from build123d import *

# Parameters (mm, degrees)
F0_R     = 8.5
F0_R_2   = 7
F1_DEPTH = 6.6
F0_R_3   = 3.1
F2_DEPTH = 9
F3_R     = 8.5
F3_R_2   = 7
F3_R_3   = 3.1
F4_DEPTH = 5
F0_R_4   = 2.6
F5_DEPTH = 6.2
F6_SIZE  = 1
F7_SIZE2 = 4
F7_SIZE  = 6
F8_SIZE  = 0.74999


# Not quite as in the source:
# - a fillet or chamfer is up to 0.001 mm smaller than in the source, because OpenCascade refuses the exact size


with BuildPart() as f1:
    # F0 (on Top) → F1 (new body)
    with BuildSketch(Plane.XY):
        Circle(F0_R)
        Circle(F0_R_2, mode=Mode.SUBTRACT)
    extrude(amount=F1_DEPTH)

    # F0 (on Top) → F2 (join)
    with BuildSketch(Plane.XY):
        Circle(F0_R_2)
        Circle(F0_R_3, mode=Mode.SUBTRACT)
    extrude(amount=F2_DEPTH)

    # F3 (on face) → F4 (join)
    with BuildSketch(Plane.XY.offset(9)):
        Circle(F3_R)
        Circle(F3_R_2, mode=Mode.SUBTRACT)
        Circle(F3_R_2)
        Circle(F3_R_3, mode=Mode.SUBTRACT)
    extrude(amount=F4_DEPTH)

    # F0 (on Top) → F5 (join)
    with BuildSketch(Plane.XY):
        Circle(F0_R_3)
        Circle(F0_R_4, mode=Mode.SUBTRACT)
    extrude(amount=F5_DEPTH)

    # F6
    f6_edges = [f1.edges().sort_by_distance(p)[0] for p in [
        (-2.6, 0, 0),
        (-8.5, 0, 0),
    ]]
    chamfer(f6_edges, length=F6_SIZE)

    # F7
    f7_edges = [f1.edges().sort_by_distance(p)[0] for p in [
        (-3.1, 0, 14),
    ]]
    f7_side = f1.faces().sort_by_distance((-3.1, 0, 10.1))[0]
    chamfer(f7_edges, length=F7_SIZE, length2=F7_SIZE2, reference=f7_side)

    # F8 (size 0.75 in the source; OpenCascade refuses exactly that, so slightly less here)
    f8_edges = [f1.edges().sort_by_distance(p)[0] for p in [
        (-7, 0, 9),
        (-7, 0, 6.6),
        (-8.5, 0, 6.6),
        (-8.5, 0, 9),
    ]]
    chamfer(f8_edges, length=F8_SIZE)


solid = f1.part
Build history of the part. All positions in model axes, mm. A direction names the side the tool comes from. Give positions to 0.01 mm unless a question says otherwise; leave off trailing zeros. Order: outer loops, then holes, each group sorted by start corner. A loop starts at its lowest first (then second) coordinate and runs counter-clockwise, first axis right, second up. Notation, with made-up numbers: M -30.5,-29.5 L -10.5,-29.5 A12 ccw -10.5,-14.5 Z; hole C -29,30 d7. An arc over 180 degrees is marked long. Put each result on its own line as item: value.
Item 1: Drop flat-ended pins along their axis: pin 1 Ø3 at (x, z) = (-3, 7.5) entering from +Y; pin 2 Ø4.5 at (x, y) = (1.5, -3) entering from -Z; pin 3 Ø5.5 at (x, y) = (0, 0) entering from +Z; pin 4 Ø8 at (y, z) = (-4.5, 5.5) entering from -X. Give the stop position or say it passes through.
Results are:
pin 1: y = 7.88
pin 2: z = 0
pin 3: z = 6.2
pin 4: x = -8.49
Item 2: Wall check: probe 1 along Y at (x, z) = (0, 2.85); probe 2 along Y at (x, z) = (0, 7.6); probe 3 along X at (y, z) = (-2.5, 11.5). Give the ranges that are in metal, low to high.
Results are:
probe 1: -8.5 to -2.6, 2.6 to 8.5
probe 2: -7 to -3.1, 3.1 to 7
probe 3: -8.12 to -4.82, 4.82 to 8.12
Item 3: Pull direction Y, two halves, no side cores. Call faces 3 (the face through (-0.338, 2.578, 3.564)), 4 (the face through (6.466, -2.681, 7.794)), 5 (the face through (-2, -7, 14)), 6 (the face through (-2, -2, 6.2)): +Y half, -Y half, draft (parallel to the pull), parting line (faces both ways), or undercut.
Results are:
face 3: undercut
face 4: parting line
face 5: draft
face 6: undercut
Item 4: Which spindle directions (+Z, -Z, +X, -X, +Y, -Y) get a long thin tool onto all of the face, cutting with end or side? Do faces 1 (the face through (4.57, 7.167, 3.391)), 2 (the face through (1.43, -2.75, 7.09)). Say none if no direction does.
Results are:
face 1: +Z, -Z
face 2: +Z
Item 5: Cut at D-D on z = 9.5. Write the cut outline in (x, y), then the cut area to 3 significant figures.
Results are:
outline: C 0,0 d16.5; hole C 0,0 d8.2
area: 161 mm2
Item 6: Cut at C-C on z = 3.25. Write the cut outline in (x, y), then the cut area to 3 significant figures.
Results are:
outline: C 0,0 d17; hole C 0,0 d5.2
area: 206 mm2
